from build123d import *

# Parameters (mm, degrees)
F0_W             = 40
F0_H             = 40
F1_DEPTH         = 2
F2_R             = 5
F3_R             = 18
F4_DEPTH         = 2
F7_R             = 2.49999
F8_R             = 0.5
F10_D            = 3
F10_COPIES_COUNT = 4


# Not quite as in the source:
# - a fillet or chamfer is up to 0.001 mm smaller than in the source, because OpenCascade refuses the exact size
# - a pattern or mirror of a feature is missing from the dataset's text; its kind, count and spacing are read off the source's solid


with BuildPart() as f1:
    # F0 (on Front) → F1 (new body)
    with BuildSketch(Plane.XZ):
        Rectangle(F0_W, F0_H)
    extrude(amount=-F1_DEPTH)

    # F2
    f2_edges = [f1.edges().sort_by_distance(p)[0] for p in [
        (20, 1, 20),
        (20, 1, -20),
        (-20, 1, -20),
        (-20, 1, 20),
    ]]
    fillet(f2_edges, radius=F2_R)

    # F3 (on face) → F4 (cut, through all)
    with BuildSketch(Plane.XZ):
        Circle(F3_R)
    extrude(amount=-F4_DEPTH, mode=Mode.SUBTRACT)

    # F5 (on Right) → F6 (revolve)
    with BuildSketch(Plane.YZ):
        with BuildLine():
            Line((18.5, 18), (0, 18))
            Line((0, 18), (-2.5, 18))
            Line((-2.5, 18), (-2.5, 13))
            Line((-2.5, 13), (0, 13))
            Line((0, 13), (4.6188021535, 5))
            Line((4.6188021535, 5), (2.6188021535, 5))
            ThreePointArc((2.6188021535, 5), (4.8290490902, 2.9220557153), (5.6443001975, 0))
            Line((5.6443001975, 0), (32.5, 0))
            Line((32.5, 0), (32.5, 13))
            Line((32.5, 13), (30.5, 13))
            Line((30.5, 13), (30.5, 15))
            Line((30.5, 15), (24.5, 15))
            Line((24.5, 15), (24.5, 13))
            Line((24.5, 13), (22.5, 13))
            Line((22.5, 13), (22.5, 14))
            Line((22.5, 14), (21.5, 14))
            Line((21.5, 14), (21.5, 15))
            Line((21.5, 15), (19.5, 15))
            Line((19.5, 15), (19.5, 14))
            Line((19.5, 14), (18.5, 14))
            Line((18.5, 14), (18.5, 18))
        make_face()
    revolve(axis=Axis((0, 19.0721500987, 0), (0, -1, 0)))

    # F7 (radius 2.5 in the source; OpenCascade refuses exactly that, so slightly less here)
    f7_edges = [f1.edges().sort_by_distance(p)[0] for p in [
        (0, -2.5, -18),
        (0, -2.5, -13),
    ]]
    fillet(f7_edges, radius=F7_R)

    # F8
    f8_edges = [f1.edges().sort_by_distance(p)[0] for p in [
        (0, 2.618802, -5),
    ]]
    fillet(f8_edges, radius=F8_R)

    # F10 (through all)
    with Locations(Plane.XZ):
        with Locations((-15, 15)):
            f10 = Hole(F10_D / 2)

    # F10_copies: F10 ×4 about axis
    f10_copies_axis = Axis((0, 0, 0), (0, 1, 0))
    for i in range(1, F10_COPIES_COUNT):
        add(f10.rotate(f10_copies_axis, i * 360 / F10_COPIES_COUNT), mode=Mode.SUBTRACT)


solid = f1.part
Here's how the part is built. I have some questions about the finished solid (model axes, mm). A direction names the side the tool comes from. Coordinates: 2 decimals unless noted, no trailing zeros. Order: outer loops, then holes, each group sorted by start corner. A loop starts at its lowest first (then second) coordinate and runs counter-clockwise, first axis right, second up. Notation, with made-up numbers: M 79.5,2.25 L 138.5,2.25 A33 cw 138.5,38.25 Z; hole C -30.75,-9 d3. An arc over 180 degrees is marked long. Answer as CSV lines item,"result".
Item 1: If I drill on line 1 (Y direction, x = -12.5, z = 6); line 2 (X direction, y = 0.05, z = 0); line 3 (Y direction, x = -11, z = 17), over which ranges is the centre line in solid material (lowest first)?
Results found:
line 1,"-1.89 to 22.5, 24.5 to 30.5"
line 2,"-20 to -12.91, 12.91 to 20"
line 3,"0 to 2"
Item 2: Imagine slicing it at B-B on y = 6.5. Write out the boundary of the cut face in (x, z).
Results found:
outline,"C 0,0 d36"
Item 3: We'd pull the mould along Y, two halves only. Please class faces 1 (the face through (0, 1, -20)), 2 (the face through (9.3, 22.5, -9.3)), 3 (the face through (-13.4, 30.5, 0.1)): +Y half, -Y half, draft (parallel to the pull), parting line (faces both ways), or undercut.
Results found:
face 1,"draft"
face 2,"undercut"
face 3,"+Y half"
Item 4: On a 3-axis mill with a long thin cutter (end or side, diameter ignored), from which of +Z, -Z, +X, -X, +Y, -Y can I reach the whole of each face in a straight line? I mean faces 4 (the face through (19, 1, 18)), 5 (the face through (-5.407, 10.134, 17.169)), 6 (the face through (-13.5, 1.01, 15.07)), 7 (the face through (-5, 0, 18)), 8 (the face through (5.362, 21.993, 12.932)). Say none if no direction works.
Results found:
face 4,"+Z, +X, +Y, -Y"
face 5,"+Y"
face 6,"+Y, -Y"
face 7,"-Y"
face 8,"none"
Item 5: Imagine slicing it at A-A on y = 25.5. Write out the boundary of the cut face in (x, z).
Results found:
outline,"C 0,0 d30"
Item 6: For pin 1 (9 mm diameter, centred on x = -3, z = 0, fed in from -Y); pin 2 (1.8 mm diameter, centred on x = 15, z = -15, fed in from +Y); pin 3 (5 mm diameter, centred on y = 28, z = 4, fed in from -X); pin 4 (3.5 mm diameter, centred on x = -15, z = 15, fed in from +Y), each with a flat end and sliding along its axis, tell me the tip position at first contact or that it passes through.
Results found:
pin 1,"y = 3.18"
pin 2,"through"
pin 3,"x = -14.92"
pin 4,"y = 2"
